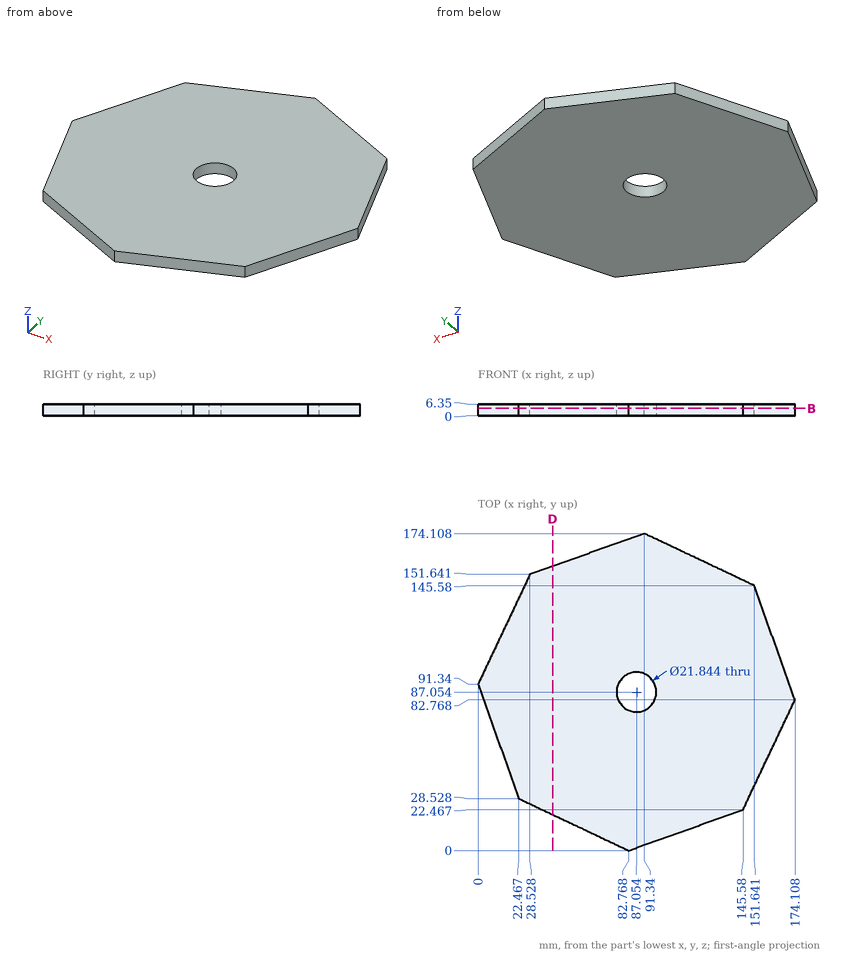
The drawing under review shows one solid part. Ordinate dimensions are in mm from its lowest x, y, z. Coordinates: 2 decimals unless noted, no trailing zeros. Write each loop counter-clockwise with the first axis right and the second up, starting at its lowest first coordinate (ties: lowest second). Pieces come first, ordered by that corner, then holes. Notation, with made-up numbers: M 84.25,33.25 L 121.25,33.25 A19 cw 121.25,67.25 Z; hole C 13.25,47.5 d8. An arc over 180 degrees is marked long. Answer as a JSON object with one key per item and string values.
Item 1: Add section B-B, the plane z = 4. Give the boundary of the cut face in (x, y) (1 decimal).
Outcome:
{"outline": "M 0,91.3 L 22.5,28.5 L 82.8,0 L 145.6,22.5 L 174.1,82.8 L 151.6,145.6 L 91.3,174.1 L 28.5,151.6 Z; hole C 87.1,87.1 d21.8"}
Item 2: Insertion check: pin 1 Ø3 at (y, z) = (123.5, 1.5) entering from -X (1 decimal); pin 2 Ø3 at (y, z) = (81, 4) entering from +X. Each pin has a flat end and moves straight along its axis. Give the tip position at first contact, or say it passes through.
Outcome:
{"pin 1": "x = 14.5", "pin 2": "x = 173.98"}
Item 3: Add section D-D, the plane x = 41. Give the boundary of the cut face in (y, z).
Outcome:
{"outline": "M 19.76,0 L 156.1,0 L 156.1,6.35 L 19.76,6.35 Z"}
Item 4: Wall thickness on probe 1 along X at (y, z) = (92, 1.5) (1 decimal); probe 2 along X at (y, z) = (44.5, 0.75) (1 decimal); probe 3 along Y at (x, z) = (57.5, 1.75) (1 decimal): over which ranges is each line inside the solid? List them lowest first.
Outcome:
{"probe 1": "0.3 to 77.3, 96.8 to 170.8", "probe 2": "16.8 to 156", "probe 3": "12 to 162"}
